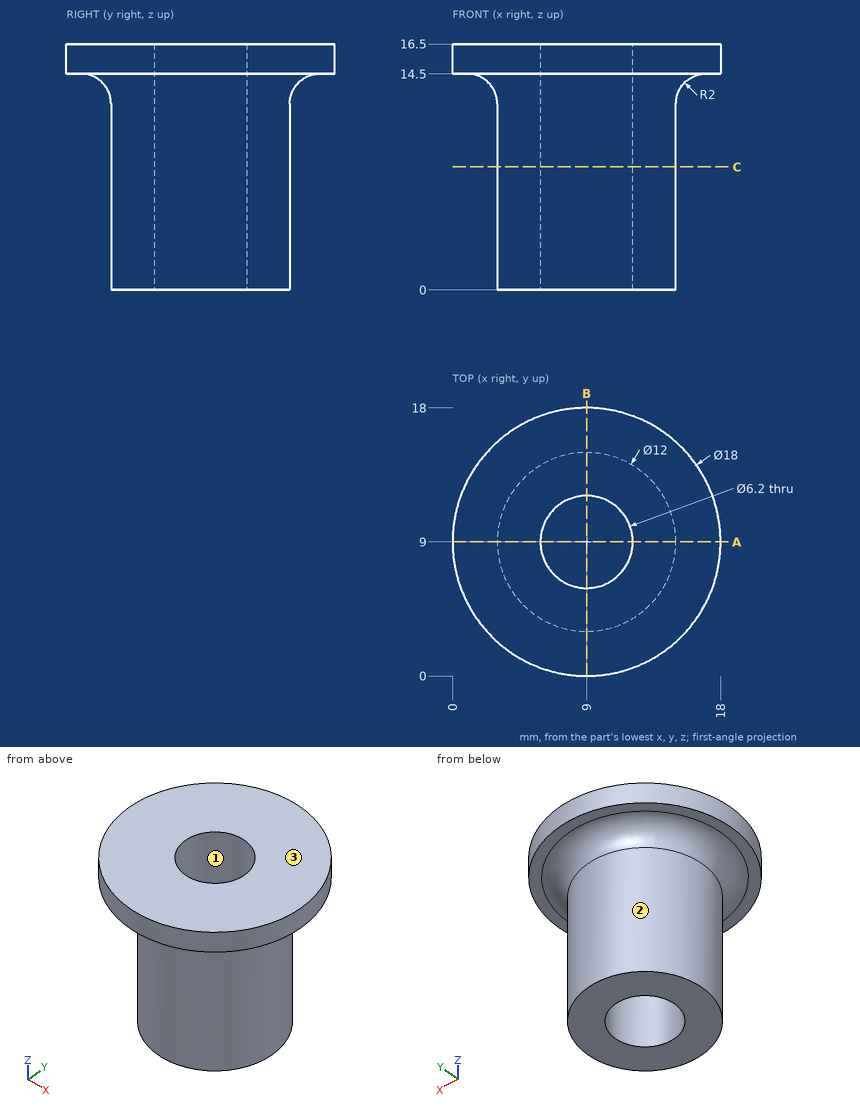
Check sheet for the drawn part. Datum: minimum x, y, z corner. Units: mm. Give positions to 0.01 mm unless a question says otherwise; leave off trailing zeros. Order: outer loops, then holes, each group sorted by start corner. A loop starts at its lowest first (then second) coordinate and runs counter-clockwise, first axis right, second up. Notation, with made-up numbers: (2, -33) -> (13, -33) arc R22 cw to (13, 3) -> close; hole circle Ø6 at (60.25, -18.5). An arc over 180 degrees is marked (long way). One line per item, written item: value.
(1) Sectioned sample at C-C on z = 8.25. Record the cut outline in (x, y), then the cut area to 3 significant figures.
Final values:
outline: circle Ø12 at (9, 9); hole circle Ø6.2 at (9, 9)
area: 82.9 mm^2
(2) Scan lines: line 1 along Y through (x, z) = (9, 5); line 2 along Z through (x, y) = (4, 2); line 3 along X through (y, z) = (7, 6). Record each from-to range of solid material in increasing order. Write a range as [from, to].
Final values:
line 1: [3, 5.9], [12.1, 15]
line 2: [14.5, 16.5]
line 3: [3.34, 6.63], [11.37, 14.66]
(3) Gauge pin test, flat ends, axial feed: pin 1 (1 mm diameter, centred on x = 12, y = 15.5, fed in from -Z); pin 2 (4 mm diameter, centred on y = 15.5, z = 6, fed in from -X); pin 3 (5 mm diameter, centred on y = 9.5, z = 10, fed in from -X). Record the tip position at first contact, or that the pin passes through.
Final values:
pin 1: z = 13.98
pin 2: x = 5.03
pin 3: x = 3
(4) Draft check along X on the marked faces 1, 2 and 3. Enter one of: pulls with the +X half, pulls with the -X half, needs draft (parallel to the pull), parting line crosses it, or undercut.
Final values:
face 1: undercut
face 2: parting line crosses it
face 3: needs draft
(5) Sectioned sample at A-A on y = 9. Record the cut outline in (x, z), then the cut area to 3 significant figures.
Final values:
outline: (0, 14.5) -> (1, 14.5) arc R2 cw to (3, 12.5) -> (3, 0) -> (5.9, 0) -> (5.9, 16.5) -> (0, 16.5) -> close; (12.1, 0) -> (15, 0) -> (15, 12.5) arc R2 cw to (17, 14.5) -> (18, 14.5) -> (18, 16.5) -> (12.1, 16.5) -> close
area: 109 mm^2
